```python
from build123d import *

# Parameters (mm, degrees)
F0_W     = 235
F0_H     = 143
F0_W_2   = 227
F0_H_2   = 128
F1_DEPTH = 5
F2_W     = 227
F2_H     = 128
F3_DEPTH = 4
F4_W     = 25
F4_H     = 20
F5_DEPTH = 20


with BuildPart() as f1:
    # F0 (on Front) → F1 (new body)
    with BuildSketch(Plane.XZ):
        with Locations((117.5, 71.5)):
            Rectangle(F0_W, F0_H)
        with Locations((116.5, 71)):
            Rectangle(F0_W_2, F0_H_2, mode=Mode.SUBTRACT)
    extrude(amount=F1_DEPTH)

    # F2 (on Front) → F3 (join)
    with BuildSketch(Plane.XZ):
        with Locations((116.5, 71)):
            Rectangle(F2_W, F2_H)
    extrude(amount=F3_DEPTH)

    # F4 (on face) → F5 (join)
    with BuildSketch(Plane(origin=(0, 0, 0), x_dir=(-1, 0, 0), z_dir=(0, 1, 0))):
        with Locations((-157.5, 20)):
            Rectangle(F4_W, F4_H)
    extrude(amount=F5_DEPTH)


solid = f1.part
```
Here's how the part is built. I have some questions about the finished solid (model axes, mm). A direction names the side the tool comes from. Give positions to 0.01 mm unless a question says otherwise; leave off trailing zeros. Write each loop counter-clockwise with the first axis right and the second up, starting at its lowest first coordinate (ties: lowest second). Pieces come first, ordered by that corner, then holes.
(1) Thinking about a two-plate mould opening in Z: for faces 1 (the face through (115, -4, 72)), 2 (the face through (158, 10, 30)), 3 (the face through (143.1, -5, 135.4)), which applies, pulls with the +Z half, pulls with the -Z half, needs draft (parallel to the pull), parting line crosses it, or undercut?
Output values:
face 1: undercut
face 2: pulls with the +Z half
face 3: needs draft
(2) Imagine slicing it at A-A, the plane x = 181.5. Write out the boundary of the cut face in (y, z).
Output values:
outline: (-5, 0) - (0, 0) - (0, 143) - (-5, 143) - (-5, 135) - (-4, 135) - (-4, 7) - (-5, 7) - close
(3) On a 3-axis mill with a long thin cutter (end or side, diameter ignored), from which of +Z, -Z, +X, -X, +Y, -Y can I reach the whole of each face in a straight line? I mean faces 4 (the face through (158, 10, 10)), 5 (the face through (170, 10, 20)), 6 (the face through (145, 10, 20)), 7 (the face through (235, -2, 70)), 8 (the face through (0, -2, 70)). Say none if no direction works.
Output values:
face 4: -Z, +X, -X, +Y
face 5: +Z, -Z, +X, +Y
face 6: +Z, -Z, -X, +Y
face 7: +Z, -Z, +X, +Y, -Y
face 8: +Z, -Z, -X, +Y, -Y
(4) Imagine slicing it at C-C, the plane y = 6. Write out the boundary of the cut face in (x, z), and give its area (3 significant figures).
Output values:
outline: (145, 10) - (170, 10) - (170, 30) - (145, 30) - close
area: 500 mm2
(5) If I drill on L1, parallel to Y at x = 111, z = 119; L2, parallel to Y at x = 211, z = 137; L3, parallel to Z at x = 167, y = 3, over which ranges is the centre line in solid material (lowest first)?
Output values:
L1: y = -4 to 0
L2: y = -5 to 0
L3: z = 10 to 30
(6) Imagine slicing it at B-B, the plane z = 126.5. Write out the boundary of the cut face in (x, y).
Output values:
outline: (0, -5) - (3, -5) - (3, -4) - (230, -4) - (230, -5) - (235, -5) - (235, 0) - (0, 0) - close
(7) Will these pins go through, and if not, where does the flat tip stop? pin 1 (6 mm diameter, centred on x = 163.5, y = 9, fed in from -Z); pin 2 (2 mm diameter, centred on x = 190.5, z = 38, fed in from +Y); pin 3 (6 mm diameter, centred on x = 39.5, z = 62.5, fed in from -Y).
Output values:
pin 1: stops at z = 10
pin 2: stops at y = 0
pin 3: stops at y = -4
